Check sheet for the drawn part. Datum: minimum x, y, z corner. Units: mm. A direction names the side the tool comes from. Round coordinates to 2 decimals unless told otherwise and drop trailing zeros. Loops run counter-clockwise (first coordinate to the right, second up) from the corner with the lowest first, then second, coordinate; pieces in that order, holes last.
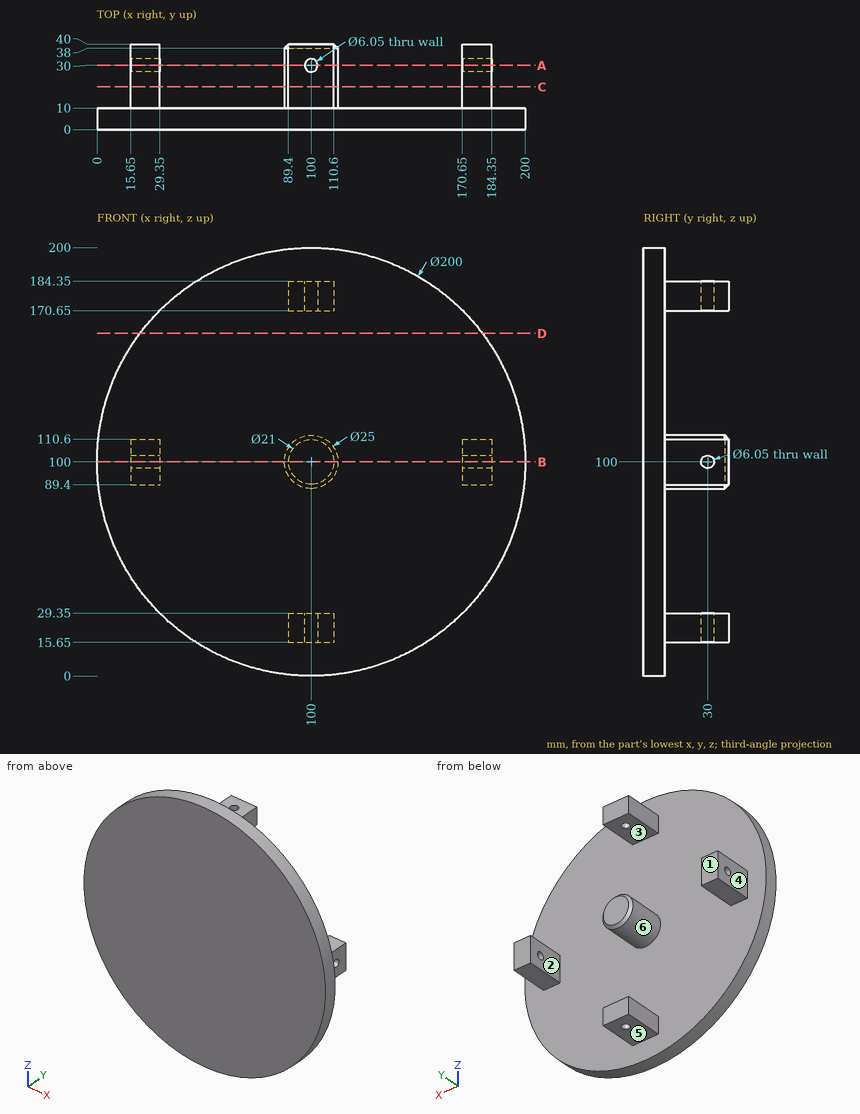
1) Scan lines: line 1 along Y through (x, z) = (100, 21.5) (3 decimals); line 2 along Z through (x, y) = (95.5, 15.5); line 3 along Z through (x, y) = (26, 17.5). Record each from-to range of solid material in increasing order.
Report:
line 1: y = 0 to 26.975, 33.025 to 40
line 2: z = 15.65 to 29.35, 88.34 to 111.66, 170.65 to 184.35
line 3: z = 89.4 to 110.6
2) Sectioned sample at C-C, the plane y = 20. Record the cut outline in (x, z), then the cut area to 3 significant figures.
Report:
outline: (15.65, 89.4) - (29.35, 89.4) - (29.35, 110.6) - (15.65, 110.6) - close; circle Ø25 at (100, 100); (89.4, 15.65) - (110.6, 15.65) - (110.6, 29.35) - (89.4, 29.35) - close; (89.4, 170.65) - (110.6, 170.65) - (110.6, 184.35) - (89.4, 184.35) - close; (170.65, 89.4) - (184.35, 89.4) - (184.35, 110.6) - (170.65, 110.6) - close
area: 1,650 mm2
3) Sectioned sample at D-D, the plane z = 160. Record the cut outline in (x, y).
Report:
outline: (20, 0) - (180, 0) - (180, 10) - (20, 10) - close
4) Sectioned sample at B-B, the plane z = 100. Record the cut outline in (x, y) (3 decimals).
Report:
outline: (0, 0) - (200, 0) - (200, 10) - (184.35, 10) - (184.35, 26.975) - (170.65, 26.975) - (170.65, 10) - (112.5, 10) - (112.5, 38) - (110.5, 40) - (89.5, 40) - (87.5, 38) - (87.5, 10) - (29.35, 10) - (29.35, 26.975) - (15.65, 26.975) - (15.65, 10) - (0, 10) - close; (15.65, 33.025) - (29.35, 33.025) - (29.35, 40) - (15.65, 40) - close; (170.65, 33.025) - (184.35, 33.025) - (184.35, 40) - (170.65, 40) - close
5) Mould release check, pull along X, two halves, no side actions. Record for the marked faces 4, 5 and 6: +X half, -X half, draft (parallel to the pull), parting line (faces both ways), or undercut.
Report:
face 4: -X half
face 5: draft
face 6: undercut
6) Gauge pin test, flat ends, axial feed: pin 1 (7 mm diameter, centred on x = 175.5, y = 28.5, fed in from -Z); pin 2 (5 mm diameter, centred on y = 30, z = 100, fed in from +X); pin 3 (17 mm diameter, centred on x = 96, y = 27.5, fed in from -Z); pin 4 (8 mm diameter, centred on x = 25, z = 40.5, fed in from -Y). Record the tip position at first contact, or that the pin passes through.
Report:
pin 1: stops at z = 89.4
pin 2: stops at x = 112.5
pin 3: stops at z = 15.65
pin 4: stops at y = 0
7) Sectioned sample at A-A, the plane y = 30. State how many separate pieces and enclosed holes the cut face has, then the cut area to 3 significant figures.
Report:
separate pieces: 9
enclosed holes: 0
area: 1,320 mm2
8) Access from +Z, -Z, +X, -X, +Y, -Y to the whole of each face (thin tool, end or side, straight path). Record for the marked faces 1, 2 and 3.
Report:
face 1: +Z, -Z, +X, -X, +Y
face 2: +Z, -Z, +Y
face 3: +X, -X, +Y
